Read the model definition and answer for the solid it produces. Units are mm, in the model's axes. Face numbers are marked on the shaded views. A direction names the side the tool comes from. Coordinates: 2 decimals unless noted, no trailing zeros. Write each loop counter-clockwise with the first axis right and the second up, starting at its lowest first coordinate (ties: lowest second). Pieces come first, ordered by that corner, then holes. Notation, with made-up numbers: (51, 1.5) -> (74, 1.5) arc R31 cw to (74, 27.5) -> close; hole circle Ø5 at (49.25, -8.75). An arc over 180 degrees is marked (long way). Write item = value, one per line. Start each with the question number.
1) Section D-D (y = -63) is taken. Determine the outline of the cut face in (x, z).
2) Section B-B (z = 8) is taken. Determine the outline of the cut face in (x, y).
3) A tool of negligible diameter and unlimited length cuts with its end or side. For the marked faces 1 and 2, from which of +Z, -Z, +X, -X, +Y, -Y can it reach the whole face along a straight path? Write none if from no direction.
4) Section C-C (x = -30.5) is taken. Determine the outline of the cut face in (y, z).
5) Flat-ended cylindrical pins translate along their axes: pin 1 Ø6 at (x, y) = (18.5, -168) entering from -Z; pin 2 Ø5 at (x, z) = (174.5, 2.5) entering from +Y; pin 3 Ø3 at (y, z) = (-163, 4) entering from -X; pin 4 Ø3 at (x, z) = (140.5, 7.5) entering from +Y. Find the tip coordinate at first contact, or state that the pin passes through.
6) Find the intervals of material crossed by line 1 along Y through (x, z) = (0, 8.5); line 2 along Y through (x, z) = (0, 2.45); line 3 along Y through (x, z) = (49, 5.5), in increasing order. Write a range as from..to.
7) Section A-A (y = -10) is taken. Determine the outline of the cut face in (x, z).
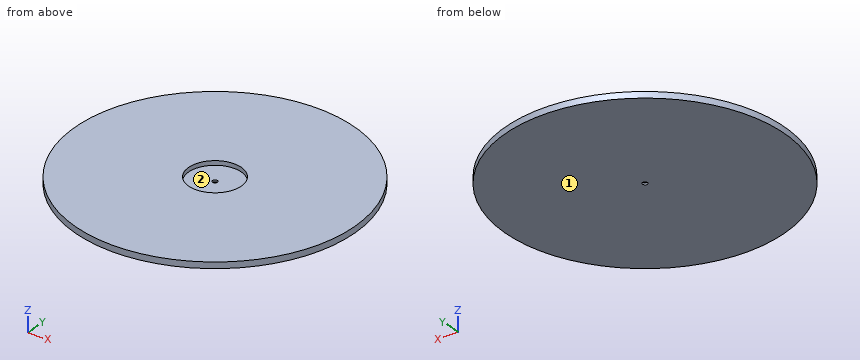
Autodesk Inventor part; units mm, degrees
ref_plane "YZ Plane" through (0, 0, 0) normal (1, 0, 0) x (0, 1, 0)
ref_plane "XZ Plane" through (0, 0, 0) normal (0, 1, 0) x (-1, 0, 0)
ref_plane "XY Plane" through (0, 0, 0) normal (0, 0, 1) x (1, 0, 0)
sketch "Sketch1" plane through (0, 0, 0) normal (0, 0, 1) x (1, 0, 0)
  circle A0 centre (0, 0) radius 225
  dimension "d0" = 450
extrude "Extrusion1" add sketch "Sketch1" along normal blind 10
sketch "Sketch2" plane through (0, 0, 10) normal (0, 0, 1) x (1, 0, 0)
  circle A0 centre (0, 0) radius 4
  dimension "d3" = 8
extrude "Extrusion2" cut sketch "Sketch2" against normal up to next
sketch "Sketch3" plane through (0, 0, 10) normal (0, 0, 1) x (1, 0, 0)
  circle A0 centre (0, 0) radius 4
  circle A1 centre (0, 0) radius 42.5
  dimension "d6" = 85
extrude "Extrusion3" cut sketch "Sketch3" against normal blind 7
properties part number "DiscoAzimute" material "Nickel-Copper Alloy 400"
Answer key:
q1.outline = (-216, 0) -> (216, 0) -> (216, 10) -> (-216, 10) -> close
q2.outline = circle Ø450 at (0, 0); hole circle Ø85 at (0, 0)
q3.face_1 = -Z, +X, -X, +Y, -Y
q3.face_2 = +Z
q4.outline = (-222.92, 0) -> (222.92, 0) -> (222.92, 10) -> (29.6, 10) -> (29.6, 3) -> (-29.6, 3) -> (-29.6, 10) -> (-222.92, 10) -> close
q5.pin_1 = 0
q5.pin_2 = 145.06
q5.pin_3 = -156.66
q5.pin_4 = 176.93
q6.line_1 = -225..-42.5, 42.5..225
q6.line_2 = -225..-4, 4..225
q6.line_3 = -219.6..219.6
q7.outline = (-224.78, 0) -> (224.78, 0) -> (224.78, 10) -> (41.31, 10) -> (41.31, 3) -> (-41.31, 3) -> (-41.31, 10) -> (-224.78, 10) -> close
